```python
from build123d import *

# Parameters (mm, degrees)
SKETCH_1_R          = 3
SKETCH_1_R_2        = 12.5
EXTRUDE_2_DEPTH     = 10
SKETCH_2_R          = 12.5
EXTRUDE_3_DEPTH     = 15
SKETCH_3_W          = 0.517195108
SKETCH_3_H          = 18.726193104
CUT_EXTRUDE_1_DEPTH = 26
SKETCH_4_R          = 2.5
CUT_EXTRUDE_2_DEPTH = 43.740275714


with BuildPart() as part:
    # 草图1 → 凸台-拉伸2 (new body)
    with BuildSketch(Plane.XY):
        with BuildLine():
            Line((-35, -7), (-7.740275714, -18.44147857))
            ThreePointArc((-7.740275714, -18.44147857), (0, -20), (7.740275714, -18.44147857))
            Line((7.740275714, -18.44147857), (35, -7))
            Line((35, -7), (35, 7))
            Line((35, 7), (7.740275714, 18.44147857))
            Line((7.740275714, 18.44147857), (7.740275714, 25.44147857))
            ThreePointArc((7.740275714, 25.44147857), (0, 27.494244152), (-7.740275714, 25.44147857))
            Line((-7.740275714, 25.44147857), (-7.740275714, 18.44147857))
            Line((-7.740275714, 18.44147857), (-35, 7))
            Line((-35, 7), (-35, -7))
        make_face()
        with Locations((-28, 0)):
            Circle(SKETCH_1_R, mode=Mode.SUBTRACT)
        Circle(SKETCH_1_R_2, mode=Mode.SUBTRACT)
        with Locations((28, 0)):
            Circle(SKETCH_1_R, mode=Mode.SUBTRACT)
    extrude(amount=EXTRUDE_2_DEPTH)

    # 草图2 → 凸台-拉伸3 (add)
    with BuildSketch(Plane.XY.offset(10)):
        with BuildLine():
            Line((-7.740275714, 18.44147857), (-7.740275714, 25.44147857))
            ThreePointArc((-7.740275714, 25.44147857), (0, 27.494244152), (7.740275714, 25.44147857))
            Line((7.740275714, 25.44147857), (7.740275714, 18.44147857))
            ThreePointArc((7.740275714, 18.44147857), (0, -20), (-7.740275714, 18.44147857))
        make_face()
        Circle(SKETCH_2_R, mode=Mode.SUBTRACT)
    extrude(amount=EXTRUDE_3_DEPTH)

    # 草图3 → 切除-拉伸1 (cut, through all)
    with BuildSketch(Plane.XY.offset(25)):
        with Locations((0, 21.741202931)):
            Rectangle(SKETCH_3_W, SKETCH_3_H)
    extrude(amount=-CUT_EXTRUDE_1_DEPTH, mode=Mode.SUBTRACT)

    # 草图4 → 切除-拉伸2 (cut, through all)
    with BuildSketch(Plane(origin=(7.740275714, 0, 0), x_dir=(0, 0, -1), z_dir=(1, 0, 0))):
        with Locations((-12.5, 21.086423576)):
            Circle(SKETCH_4_R)
    extrude(amount=-CUT_EXTRUDE_2_DEPTH, mode=Mode.SUBTRACT)


solid = part.part
```
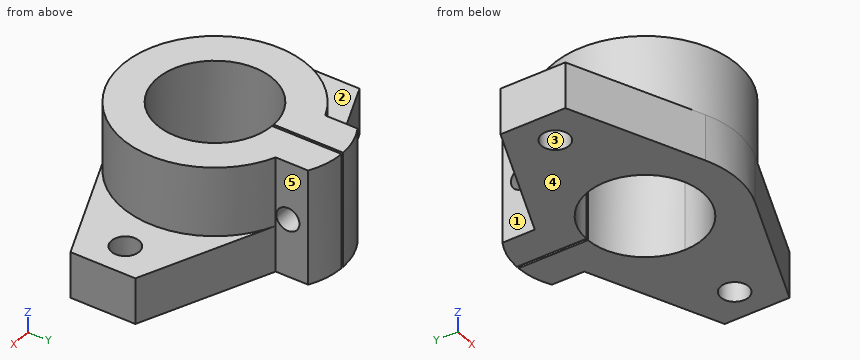
Input: part model. Units: mm. Frame: model coordinates. Face numbers are marked on the shaded views. A direction names the side the tool comes from. Coordinates: 2 decimals unless noted, no trailing zeros. Write each loop counter-clockwise with the first axis right and the second up, starting at its lowest first coordinate (ties: lowest second). Pieces come first, ordered by that corner, then holes.
1) Mould query, pull axis X, two halves, no side actions, for the marked faces 1, 2 and 3. Classes: pulls with the +X half, pulls with the -X half, needs draft (parallel to the pull), parting line crosses it, or undercut.
2) Section A-A on z = 12.5. Output: boundary loops of the cut face in (x, y), and give its area (3 significant figures).
3) Section C-C on y = -10.5. Output: boundary loops of the cut face in (x, z), and give its area (3 significant figures).
4) Material intervals for line 1 along X through (y, z) = (0.5, 12); line 2 along X through (y, z) = (20.5, 22.75); line 3 along Y through (x, z) = (4.5, 13.5), sorted ascending.
5) Set-up query: the marked faces 4 and 5. Return all of +Z, -Z, +X, -X, +Y, -Y with unobstructed straight access to the full face (end or side cutting, diameter ignored); none if empty.
6) Section B-B on x = 4. Output: boundary loops of the cut face in (y, z).
7) Section D-D on x = 28. Output: boundary loops of the cut face in (y, z).
8) Pin query (flat end, axial travel): pin 1 Ø7 at (x, y) = (28, 0) entering from +Z; pin 2 Ø12 at (y, z) = (-14, 9.5) entering from -X; pin 3 Ø1.5 at (x, z) = (-19.5, 3.5) entering from -Y. Return the tip coordinate at first contact, or that it passes through.
Check result:
1. face 1: pulls with the -X half
1. face 2: needs draft
1. face 3: undercut
2. outline: (-7.74, 18.44) arc R20 ccw (long way) to (7.74, 18.44) - (7.74, 18.59) - (0.26, 18.59) - (0.26, 12.5) arc R12.5 cw (long way) to (-0.26, 12.5) - (-0.26, 18.59) - (-7.74, 18.59) - close; (-7.74, 23.59) - (-0.26, 23.59) - (-0.26, 27.49) arc R15.62 ccw to (-7.74, 25.44) - close; (0.26, 23.59) - (7.74, 23.59) - (7.74, 25.44) arc R15.62 ccw to (0.26, 27.49) - close
2. area: 797 mm2
3. outline: (-26.66, 0) - (-6.78, 0) - (-6.78, 25) - (-17.02, 25) - (-17.02, 10) - (-26.66, 10) - close; (6.78, 0) - (26.66, 0) - (26.66, 10) - (17.02, 10) - (17.02, 25) - (6.78, 25) - close
3. area: 705 mm2
4. line 1: x = -19.99 to -12.49, 12.49 to 19.99
4. line 2: x = -7.74 to -0.26, 0.26 to 7.74
4. line 3: y = -19.49 to -11.66, 11.66 to 18.8, 23.38 to 26.83
5. face 4: -Z, +X, -X, +Y, -Y
5. face 5: +Z, -Z, +X, +Y
6. outline: (-19.6, 0) - (-11.84, 0) - (-11.84, 25) - (-19.6, 25) - close; (11.84, 0) - (26.97, 0) - (26.97, 25) - (11.84, 25) - close; hole circle Ø5 at (21.09, 12.5)
7. outline: (-9.94, 0) - (-3, 0) - (-3, 10) - (-9.94, 10) - close; (3, 0) - (9.94, 0) - (9.94, 10) - (3, 10) - close
8. pin 1: stops at z = 10
8. pin 2: stops at x = -32.62
8. pin 3: stops at y = -13.82
